Build history of the part. All positions in model axes, mm. A direction names the side the tool comes from. Round coordinates to 2 decimals unless told otherwise and drop trailing zeros. Order: outer loops, then holes, each group sorted by start corner. A loop starts at its lowest first (then second) coordinate and runs counter-clockwise, first axis right, second up. Notation, with made-up numbers: (-25, -3) -> (-7, -3) arc R10 ccw to (-7, 1) -> close; hole circle Ø5 at (45.25, -35). An arc over 180 degrees is marked (long way). Answer as a JSON object with one key per item and string values.
from build123d import *

# Parameters (mm, degrees)
SKETCH_1_W                   = 88.39
SKETCH_1_H                   = 150
EXTRUDE_1_DEPTH              = 5
SKETCH_2_R                   = 7.5
EXTRUDE_2_DEPTH              = 15
HOLE_WIZARD_1_D              = 8
EXTRUDE_3_DEPTH              = 15
SKETCH_8_R                   = 4
CUT_EXTRUDE_1_DEPTH          = 166.891205614
HOLE_WIZARD_M3_1_D           = 3.2
HOLE_WIZARD_M3_1_CSINK_D     = 3.45
HOLE_WIZARD_M3_1_CSINK_ANGLE = 90


with BuildPart() as part:
    # 스케치1 → 보스-돌출1 (new body)
    with BuildSketch(Plane.XY):
        with Locations((44.195, 75)):
            Rectangle(SKETCH_1_W, SKETCH_1_H)
    extrude(amount=EXTRUDE_1_DEPTH)

    # 스케치2 → 보스-돌출2 (add)
    with BuildSketch(Plane(origin=(0, 150, 0), x_dir=(1, 0, 0), z_dir=(0, 1, 0))):
        with Locations((88.39, -2.5)):
            Circle(SKETCH_2_R)
        with Locations((0, -2.5)):
            Circle(SKETCH_2_R)
    extrude(amount=-EXTRUDE_2_DEPTH)

    # 구멍1 (through all)
    with Locations(Plane(origin=(0, 150, 0), x_dir=(1, 0, 0), z_dir=(0, 1, 0))):
        with Locations((0, -2.5), (88.39, -2.5)):
            Hole(HOLE_WIZARD_1_D / 2)

    # 스케치7 → 보스-돌출3 (add)
    with BuildSketch(Plane.XZ):
        with BuildLine():
            Line((81.318932188, 0), (85.267501001, 0))
            ThreePointArc((85.267501001, 0), (84.39, 2.5), (85.267501001, 5))
            Line((85.267501001, 5), (81.318932188, 5))
            ThreePointArc((81.318932188, 5), (95.89, 2.5), (81.318932188, 0))
        make_face()
        with BuildLine():
            Line((3.122498999, 5), (7.071067812, 5))
            ThreePointArc((7.071067812, 5), (-7.5, 2.5), (7.071067812, 0))
            Line((7.071067812, 0), (3.122498999, 0))
            ThreePointArc((3.122498999, 0), (4, 2.5), (3.122498999, 5))
        make_face()
    extrude(amount=-EXTRUDE_3_DEPTH)

    # 스케치8 → 컷-돌출1 (cut, through all)
    with BuildSketch(Plane(origin=(0, 15, 0), x_dir=(1, 0, 0), z_dir=(0, 1, 0))):
        with Locations(Location((0, -2.5, 0), (0, 0, 270))):
            Circle(SKETCH_8_R)
        with Locations(Location((88.39, -2.5, 0), (0, 0, 270))):
            Circle(SKETCH_8_R)
    extrude(amount=-CUT_EXTRUDE_1_DEPTH, mode=Mode.SUBTRACT)

    # M3 여유 구멍1 (through all)
    with Locations(Plane.XY.offset(5)):
        with Locations((41.222498999, 73.8), (28.522498999, 48.4)):
            CounterSinkHole(HOLE_WIZARD_M3_1_D / 2, HOLE_WIZARD_M3_1_CSINK_D / 2, counter_sink_angle=HOLE_WIZARD_M3_1_CSINK_ANGLE)


solid = part.part
1) Which spindle directions (+Z, -Z, +X, -X, +Y, -Y) get a long thin tool onto all of the face, cutting with end or side? Do faces 1 (the face through (92, 135, 6)), 2 (the face through (41.431, 75.386, 2.403)). Say none if no direction does.
Checked values:
{"face 1": "+X", "face 2": "+Z, -Z"}
2) Cut at B-B, the plane z = 2.5. Give the cut face in (x, y).
Checked values:
{"outline": "(-7.5, 0) -> (-4, 0) -> (-4, 15) -> (-7.5, 15) -> close; (-7.5, 135) -> (-4, 135) -> (-4, 150) -> (-7.5, 150) -> close; (4, 0) -> (84.39, 0) -> (84.39, 150) -> (4, 150) -> close; (92.39, 0) -> (95.89, 0) -> (95.89, 15) -> (92.39, 15) -> close; (92.39, 135) -> (95.89, 135) -> (95.89, 150) -> (92.39, 150) -> close; hole circle Ø3.2 at (28.52, 48.4); hole circle Ø3.2 at (41.22, 73.8)"}
3) Cut at D-D, the plane y = 17.5. Give the cut face in (x, z).
Checked values:
{"outline": "(3.12, 0) -> (85.27, 0) arc R4 cw to (85.27, 5) -> (3.12, 5) arc R4 cw to start"}
4) Cut at C-C, the plane x = 88.39. Give the cut face in (y, z), plus the area to 3 significant figures.
Checked values:
{"outline": "(0, -5) -> (15, -5) -> (15, -1.5) -> (0, -1.5) -> close; (0, 6.5) -> (15, 6.5) -> (15, 10) -> (0, 10) -> close; (135, -5) -> (150, -5) -> (150, -1.5) -> (135, -1.5) -> close; (135, 6.5) -> (150, 6.5) -> (150, 10) -> (135, 10) -> close", "area": "210 mm²"}
5) Pull direction Y, two halves, no side cores. Call faces 3 (the face through (30.12, 48.47, 2.4)), 4 (the face through (-7.494, 7.395, 2.794)), 5 (the face through (43, 150, 2)): pulls with the +Y half, pulls with the -Y half, needs draft (parallel to the pull), parting line crosses it, or undercut.
Checked values:
{"face 3": "undercut", "face 4": "needs draft", "face 5": "pulls with the +Y half"}
6) Probe L1, parallel to X at y = 9.75, z = 2.5; L2, parallel to Y at x = 85.5, z = 9; L3, parallel to X at y = 73.8, z = 2.1. List the from-to ranges inside material, lowest first. Write a range as from..to.
Checked values:
{"L1": "x = -7.5..-4, 4..84.39, 92.39..95.89", "L2": "y = 0..15, 135..150", "L3": "x = 3.98..39.62, 42.82..84.41"}
7) Flat gauge pins, fed straight in: pin 1 Ø4 at (x, y) = (28.52, 48.4) entering from +Z; pin 2 Ø3 at (x, y) = (41.22, 73.8) entering from +Z; pin 3 Ø4.5 at (x, z) = (90.5, -1) entering from -Y; pin 4 Ø3 at (y, z) = (78.5, 0.5) entering from -X. Where does each tip first touch, or does it go through?
Checked values:
{"pin 1": "stops at z = 5", "pin 2": "passes through", "pin 3": "stops at y = 0", "pin 4": "stops at x = 3.12"}
